from build123d import *

# Parameters (mm, degrees)
ESQUISSE1_R      = 14.25
ESQUISSE1_R_2    = 2.25
EXTRUSION1_DEPTH = 2


with BuildPart() as part:
    # Esquisse1 → Extrusion1 (new body)
    with BuildSketch(Plane(origin=(0, 0, 0), x_dir=(1, 0, 0), z_dir=(0, 1, 0))):
        with BuildLine():
            Line((13.533333333, 16.057673832), (26.688888889, 4.970232377))
            ThreePointArc((26.688888889, 4.970232377), (29, 0), (26.688888889, -4.970232377))
            Line((26.688888889, -4.970232377), (13.533333333, -16.057673832))
            ThreePointArc((13.533333333, -16.057673832), (0, -21), (-13.533333333, -16.057673832))
            Line((-13.533333333, -16.057673832), (-26.688888889, -4.970232377))
            ThreePointArc((-26.688888889, -4.970232377), (-29, 0), (-26.688888889, 4.970232377))
            Line((-26.688888889, 4.970232377), (-13.533333333, 16.057673832))
            ThreePointArc((-13.533333333, 16.057673832), (0, 21), (13.533333333, 16.057673832))
        make_face()
        with Locations(Location((0, 0, 0), (0, 0, 270))):
            Circle(ESQUISSE1_R, mode=Mode.SUBTRACT)
        with Locations(Location((22.5, 0, 0), (0, 0, 270))):
            Circle(ESQUISSE1_R_2, mode=Mode.SUBTRACT)
        with Locations(Location((-22.5, 0, 0), (0, 0, 270))):
            Circle(ESQUISSE1_R_2, mode=Mode.SUBTRACT)
    extrude(amount=EXTRUSION1_DEPTH)


solid = part.part
The model under review builds one solid part; all positions refer to its coordinate system, in mm. Coordinates: 2 decimals unless noted, no trailing zeros. Write each loop counter-clockwise with the first axis right and the second up, starting at its lowest first coordinate (ties: lowest second). Pieces come first, ordered by that corner, then holes. Notation, with made-up numbers: (35, 70.5) - (59, 70.5) arc R13 cw to (59, 80.5) - close; hole circle Ø10 at (78.25, 59.5). An arc over 180 degrees is marked (long way). Answer as a JSON object with one key per item and string values. Group by question number.
1. Clearance check with flat-ended pins moving along their axes: pin 1 Ø2.5 at (x, z) = (-22.5, 0) entering from -Y; pin 2 Ø1 at (x, y) = (23, 1.5) entering from -Z; pin 3 Ø1 at (x, y) = (-5, 1.5) entering from -Z; pin 4 Ø1 at (y, z) = (1, 6.5) entering from +X. State where each tip first meets the part, or that it passes through.
2. Add section C-C (z = -1.5). Give the boundary of the cut face in (x, y), plus the area to 3 significant figures.
3. Add section A-A (y = 0.85). Give the boundary of the cut face in (x, z).
4. To check wall thickness, follow probe 1 along X at (y, z) = (0.4, 0); probe 2 along Z at (x, y) = (6.5, 1.65); probe 3 along Z at (x, y) = (-21, 1). State the ranges of each line that lie inside material, in increasing order.
5. Add section D-D (z = -9). Give the boundary of the cut face in (x, y).
6. Add section B-B (x = 0). Give the boundary of the cut face in (y, z).
7. Mouldability with a two-part tool opening along X and no side actions: class faces 1 (the face through (-29, 1, 0)), 2 (the face through (20.02, 0.99, -10.59)), 3 (the face through (20.304, 0.986, -0.488)) as pulls with the +X half, pulls with the -X half, needs draft (parallel to the pull), parting line crosses it, or undercut.
Findings:
{
 "1": {"pin 1": "through", "pin 2": "z = -8.5", "pin 3": "z = -20.51", "pin 4": "x = 25.47"},
 "2": {"outline": "(-28.82, 0) - (-24.18, 0) - (-24.18, 2) - (-28.82, 2) - close; (-20.82, 0) - (-14.17, 0) - (-14.17, 2) - (-20.82, 2) - close; (14.17, 0) - (20.82, 0) - (20.82, 2) - (14.17, 2) - close; (24.18, 0) - (28.82, 0) - (28.82, 2) - (24.18, 2) - close", "area": "45.2 mm²"},
 "3": {"outline": "(-26.69, -4.97) - (-13.53, -16.06) arc R21 ccw to (13.53, -16.06) - (26.69, -4.97) arc R6.5 ccw to (26.69, 4.97) - (13.53, 16.06) arc R21 ccw to (-13.53, 16.06) - (-26.69, 4.97) arc R6.5 ccw to start; hole circle Ø4.5 at (-22.5, 0); hole circle Ø28.5 at (0, 0); hole circle Ø4.5 at (22.5, 0)"},
 "4": {"probe 1": "-29 to -24.75, -20.25 to -14.25, 14.25 to 20.25, 24.75 to 29", "probe 2": "-19.97 to -12.68, 12.68 to 19.97", "probe 3": "-9.76 to -1.68, 1.68 to 9.76"},
 "5": {"outline": "(-21.91, 0) - (-11.05, 0) - (-11.05, 2) - (-21.91, 2) - close; (11.05, 0) - (21.91, 0) - (21.91, 2) - (11.05, 2) - close"},
 "6": {"outline": "(0, -21) - (2, -21) - (2, -14.25) - (0, -14.25) - close; (0, 14.25) - (2, 14.25) - (2, 21) - (0, 21) - close"},
 "7": {"face 1": "pulls with the -X half", "face 2": "pulls with the +X half", "face 3": "undercut"}
}
